```python
from build123d import *

# Parameters (mm, degrees)
F0_R     = 5
F0_R_2   = 3.15
F0_R_3   = 2.55
F1_DEPTH = 3.25
F2_R     = 2.55
F3_DEPTH = 14


# Not quite as in the source:
# - a feature names something its author has since deleted; it is built from what else it names


with BuildPart() as f1:
    # F0 (on Top) → F1 (new body)
    with BuildSketch(Plane.XY):
        with BuildLine():
            Line((-5.95, -4.4), (-4.4034787385, -4.4))
            ThreePointArc((-4.4034787385, -4.4), (0, -6.225), (4.4034787385, -4.4))
            Line((4.4034787385, -4.4), (5.95, -4.4))
            Line((5.95, -4.4), (5.95, 4.4))
            Line((5.95, 4.4), (4.4034787385, 4.4))
            ThreePointArc((4.4034787385, 4.4), (0, 6.225), (-4.4034787385, 4.4))
            Line((-4.4034787385, 4.4), (-5.95, 4.4))
            Line((-5.95, 4.4), (-5.95, -4.4))
        make_face()
        Circle(F0_R, mode=Mode.SUBTRACT)
        Circle(F0_R)
        Circle(F0_R_2, mode=Mode.SUBTRACT)
        Circle(F0_R_2)
        Circle(F0_R_3, mode=Mode.SUBTRACT)
        Circle(F0_R_3)
        with BuildLine():
            ThreePointArc((-1.275, -1.1244443072), (-0.601040764, 1.5902043894), (1.7, 0))
            ThreePointArc((1.7, 0), (1.5902043894, -0.601040764), (1.275, -1.1244443072))
            ThreePointArc((1.275, -1.1244443072), (0, -1.7), (-1.275, -1.1244443072))
        make_face(mode=Mode.SUBTRACT)
        with BuildLine():
            Line((1.275, -1.1244443072), (-1.275, -1.1244443072))
            ThreePointArc((-1.275, -1.1244443072), (0, -1.7), (1.275, -1.1244443072))
        make_face()
    extrude(amount=F1_DEPTH)

    # F2 (on face) → F3 (join)
    with BuildSketch(Plane.XY.offset(3.25)):
        with BuildLine():
            ThreePointArc((-4.8302633262, 0.3000085552), (-4.9546244936, 0.172348246), (-5, 0))
            ThreePointArc((-5, 0), (-4.9546244936, -0.172348246), (-4.8302633262, -0.3000085552))
            Line((-4.8302633262, -0.3000085552), (-4.2601369618, -0.6425750355))
            ThreePointArc((-4.2601369618, -0.6425750355), (-4.0929165173, -0.7205512094), (-3.9131380826, -0.7620563314))
            Line((-3.9131380826, -0.7620563314), (-3.3117988826, -0.835891501))
            ThreePointArc((-3.3117988826, -0.835891501), (-3.0868883315, -0.9291389359), (-2.9422567869, -1.125))
            ThreePointArc((-2.9422567869, -1.125), (-3.15, 0), (-2.9422567869, 1.125))
            ThreePointArc((-2.9422567869, 1.125), (-3.0868883315, 0.9291389359), (-3.3117988826, 0.835891501))
            Line((-3.3117988826, 0.835891501), (-3.9131380826, 0.7620563314))
            ThreePointArc((-3.9131380826, 0.7620563314), (-4.0929165173, 0.7205512094), (-4.2601369618, 0.6425750355))
            Line((-4.2601369618, 0.6425750355), (-4.8302633262, 0.3000085552))
        make_face()
        with BuildLine():
            ThreePointArc((-3.2033738691, 3.6276500367), (-3.3815799641, 3.6253171911), (-3.5355339059, 3.5355339059))
            ThreePointArc((-3.5355339059, 3.5355339059), (-3.6253171911, 3.3815799641), (-3.6276500367, 3.2033738691))
            Line((-3.6276500367, 3.2033738691), (-3.4667408995, 2.5580025694))
            ThreePointArc((-3.4667408995, 2.5580025694), (-3.4036356706, 2.3846223779), (-3.3058616735, 2.2281512744))
            Line((-3.3058616735, 2.2281512744), (-2.9328599965, 1.7507308991))
            ThreePointArc((-2.9328599965, 1.7507308991), (-2.8397601142, 1.5257592297), (-2.8759848548, 1.2849945972))
            ThreePointArc((-2.8759848548, 1.2849945972), (-2.2273863607, 2.2273863607), (-1.2849945972, 2.8759848548))
            ThreePointArc((-1.2849945972, 2.8759848548), (-1.5257592297, 2.8397601142), (-1.7507308991, 2.9328599965))
            Line((-1.7507308991, 2.9328599965), (-2.2281512744, 3.3058616735))
            ThreePointArc((-2.2281512744, 3.3058616735), (-2.3846223779, 3.4036356706), (-2.5580025694, 3.4667408995))
            Line((-2.5580025694, 3.4667408995), (-3.2033738691, 3.6276500367))
        make_face()
        with BuildLine():
            ThreePointArc((0.3000085552, 4.8302633262), (0.172348246, 4.9546244936), (0, 5))
            ThreePointArc((0, 5), (-0.172348246, 4.9546244936), (-0.3000085552, 4.8302633262))
            Line((-0.3000085552, 4.8302633262), (-0.6425750355, 4.2601369618))
            ThreePointArc((-0.6425750355, 4.2601369618), (-0.7205512094, 4.0929165173), (-0.7620563314, 3.9131380826))
            Line((-0.7620563314, 3.9131380826), (-0.835891501, 3.3117988826))
            ThreePointArc((-0.835891501, 3.3117988826), (-0.9291389359, 3.0868883315), (-1.125, 2.9422567869))
            ThreePointArc((-1.125, 2.9422567869), (0, 3.15), (1.125, 2.9422567869))
            ThreePointArc((1.125, 2.9422567869), (0.9291389359, 3.0868883315), (0.835891501, 3.3117988826))
            Line((0.835891501, 3.3117988826), (0.7620563314, 3.9131380826))
            ThreePointArc((0.7620563314, 3.9131380826), (0.7205512094, 4.0929165173), (0.6425750355, 4.2601369618))
            Line((0.6425750355, 4.2601369618), (0.3000085552, 4.8302633262))
        make_face()
        with BuildLine():
            ThreePointArc((3.2033738691, -3.6276500367), (3.3815799667, -3.6253171904), (3.5355339096, -3.5355339023))
            ThreePointArc((3.5355339096, -3.5355339023), (3.6253171918, -3.3815799616), (3.6276500367, -3.2033738691))
            Line((3.6276500367, -3.2033738691), (3.4667408995, -2.5580025694))
            ThreePointArc((3.4667408995, -2.5580025694), (3.4036356706, -2.3846223779), (3.3058616735, -2.2281512744))
            Line((3.3058616735, -2.2281512744), (2.9328599965, -1.7507308991))
            ThreePointArc((2.9328599965, -1.7507308991), (2.8397601142, -1.5257592297), (2.8759848548, -1.2849945972))
            ThreePointArc((2.8759848548, -1.2849945972), (2.2273863607, -2.2273863607), (1.2849945972, -2.8759848548))
            ThreePointArc((1.2849945972, -2.8759848548), (1.5257592297, -2.8397601142), (1.7507308991, -2.9328599965))
            Line((1.7507308991, -2.9328599965), (2.2281512744, -3.3058616735))
            ThreePointArc((2.2281512744, -3.3058616735), (2.3846223779, -3.4036356706), (2.5580025694, -3.4667408995))
            Line((2.5580025694, -3.4667408995), (3.2033738691, -3.6276500367))
        make_face()
        with BuildLine():
            ThreePointArc((-0.3000085552, -4.8302633262), (-0.172348246, -4.9546244936), (0, -5))
            ThreePointArc((0, -5), (0.172348246, -4.9546244936), (0.3000085552, -4.8302633262))
            Line((0.3000085552, -4.8302633262), (0.6425750355, -4.2601369618))
            ThreePointArc((0.6425750355, -4.2601369618), (0.7205512094, -4.0929165173), (0.7620563314, -3.9131380826))
            Line((0.7620563314, -3.9131380826), (0.835891501, -3.3117988826))
            ThreePointArc((0.835891501, -3.3117988826), (0.9291389359, -3.0868883315), (1.125, -2.9422567869))
            ThreePointArc((1.125, -2.9422567869), (0, -3.15), (-1.125, -2.9422567869))
            ThreePointArc((-1.125, -2.9422567869), (-0.9291389359, -3.0868883315), (-0.835891501, -3.3117988826))
            Line((-0.835891501, -3.3117988826), (-0.7620563314, -3.9131380826))
            ThreePointArc((-0.7620563314, -3.9131380826), (-0.7205512094, -4.0929165173), (-0.6425750355, -4.2601369618))
            Line((-0.6425750355, -4.2601369618), (-0.3000085552, -4.8302633262))
        make_face()
        with BuildLine():
            ThreePointArc((-3.6276500367, -3.2033738691), (-3.6253171911, -3.3815799641), (-3.5355339059, -3.5355339059))
            ThreePointArc((-3.5355339059, -3.5355339059), (-3.3815799641, -3.6253171911), (-3.2033738691, -3.6276500367))
            Line((-3.2033738691, -3.6276500367), (-2.5580025694, -3.4667408995))
            ThreePointArc((-2.5580025694, -3.4667408995), (-2.3846223779, -3.4036356706), (-2.2281512744, -3.3058616735))
            Line((-2.2281512744, -3.3058616735), (-1.7507308991, -2.9328599965))
            ThreePointArc((-1.7507308991, -2.9328599965), (-1.5257592297, -2.8397601142), (-1.2849945972, -2.8759848548))
            ThreePointArc((-1.2849945972, -2.8759848548), (-2.2273863607, -2.2273863607), (-2.8759848548, -1.2849945972))
            ThreePointArc((-2.8759848548, -1.2849945972), (-2.8397601142, -1.5257592297), (-2.9328599965, -1.7507308991))
            Line((-2.9328599965, -1.7507308991), (-3.3058616735, -2.2281512744))
            ThreePointArc((-3.3058616735, -2.2281512744), (-3.4036356706, -2.3846223779), (-3.4667408995, -2.5580025694))
            Line((-3.4667408995, -2.5580025694), (-3.6276500367, -3.2033738691))
        make_face()
        with BuildLine():
            ThreePointArc((2.8759848548, -1.2849945972), (2.9102205274, -1.205452812), (2.9422567869, -1.125))
            ThreePointArc((2.9422567869, -1.125), (3.0976288414, -0.5720101054), (3.15, 0))
            ThreePointArc((3.15, 0), (3.0976288414, 0.5720101054), (2.9422567869, 1.125))
            ThreePointArc((2.9422567869, 1.125), (2.9102205274, 1.205452812), (2.8759848548, 1.2849945972))
            ThreePointArc((2.8759848548, 1.2849945972), (2.2273863607, 2.2273863607), (1.2849945972, 2.8759848548))
            ThreePointArc((1.2849945972, 2.8759848548), (1.205452812, 2.9102205274), (1.125, 2.9422567869))
            ThreePointArc((1.125, 2.9422567869), (0, 3.15), (-1.125, 2.9422567869))
            ThreePointArc((-1.125, 2.9422567869), (-1.205452812, 2.9102205274), (-1.2849945972, 2.8759848548))
            ThreePointArc((-1.2849945972, 2.8759848548), (-2.2273863607, 2.2273863607), (-2.8759848548, 1.2849945972))
            ThreePointArc((-2.8759848548, 1.2849945972), (-2.9102205274, 1.205452812), (-2.9422567869, 1.125))
            ThreePointArc((-2.9422567869, 1.125), (-3.15, 0), (-2.9422567869, -1.125))
            ThreePointArc((-2.9422567869, -1.125), (-2.9102205274, -1.205452812), (-2.8759848548, -1.2849945972))
            ThreePointArc((-2.8759848548, -1.2849945972), (-2.2273863607, -2.2273863607), (-1.2849945972, -2.8759848548))
            ThreePointArc((-1.2849945972, -2.8759848548), (-1.205452812, -2.9102205274), (-1.125, -2.9422567869))
            ThreePointArc((-1.125, -2.9422567869), (0, -3.15), (1.125, -2.9422567869))
            ThreePointArc((1.125, -2.9422567869), (1.205452812, -2.9102205274), (1.2849945972, -2.8759848548))
            ThreePointArc((1.2849945972, -2.8759848548), (2.2273863607, -2.2273863607), (2.8759848548, -1.2849945972))
        make_face()
        Circle(F2_R, mode=Mode.SUBTRACT)
        Circle(F2_R)
        with BuildLine():
            Line((1.275, -1.1244443072), (-1.275, -1.1244443072))
            ThreePointArc((-1.275, -1.1244443072), (0, 1.7), (1.275, -1.1244443072))
        make_face(mode=Mode.SUBTRACT)
        with BuildLine():
            ThreePointArc((3.6276500367, 3.2033738691), (3.6253171915, 3.3815799629), (3.5355339078, 3.5355339041))
            ThreePointArc((3.5355339078, 3.5355339041), (3.3815799654, 3.6253171908), (3.2033738691, 3.6276500367))
            Line((3.2033738691, 3.6276500367), (2.5580025694, 3.4667408995))
            ThreePointArc((2.5580025694, 3.4667408995), (2.3846223779, 3.4036356706), (2.2281512744, 3.3058616735))
            Line((2.2281512744, 3.3058616735), (1.7507308991, 2.9328599965))
            ThreePointArc((1.7507308991, 2.9328599965), (1.5257592297, 2.8397601142), (1.2849945972, 2.8759848548))
            ThreePointArc((1.2849945972, 2.8759848548), (2.2273863607, 2.2273863607), (2.8759848548, 1.2849945972))
            ThreePointArc((2.8759848548, 1.2849945972), (2.8397601142, 1.5257592297), (2.9328599965, 1.7507308991))
            Line((2.9328599965, 1.7507308991), (3.3058616735, 2.2281512744))
            ThreePointArc((3.3058616735, 2.2281512744), (3.4036356706, 2.3846223779), (3.4667408995, 2.5580025694))
            Line((3.4667408995, 2.5580025694), (3.6276500367, 3.2033738691))
        make_face()
        with BuildLine():
            ThreePointArc((4.8302633262, -0.3000085552), (4.9546244936, -0.172348246), (5, 0))
            ThreePointArc((5, 0), (4.9546244936, 0.172348246), (4.8302633262, 0.3000085552))
            Line((4.8302633262, 0.3000085552), (4.2601369618, 0.6425750355))
            ThreePointArc((4.2601369618, 0.6425750355), (4.0929165173, 0.7205512094), (3.9131380826, 0.7620563314))
            Line((3.9131380826, 0.7620563314), (3.3117988826, 0.835891501))
            ThreePointArc((3.3117988826, 0.835891501), (3.0868883315, 0.9291389359), (2.9422567869, 1.125))
            ThreePointArc((2.9422567869, 1.125), (3.0976288414, 0.5720101054), (3.15, 0))
            ThreePointArc((3.15, 0), (3.0976288414, -0.5720101054), (2.9422567869, -1.125))
            ThreePointArc((2.9422567869, -1.125), (3.0868883315, -0.9291389359), (3.3117988826, -0.835891501))
            Line((3.3117988826, -0.835891501), (3.9131380826, -0.7620563314))
            ThreePointArc((3.9131380826, -0.7620563314), (4.0929165173, -0.7205512094), (4.2601369618, -0.6425750355))
            Line((4.2601369618, -0.6425750355), (4.8302633262, -0.3000085552))
        make_face()
    extrude(amount=F3_DEPTH)


solid = f1.part
```
Geometry check sheet. Reference: the model listing, model coordinates, mm. A direction names the side the tool comes from. Round coordinates to 2 decimals unless told otherwise and drop trailing zeros. Order: outer loops, then holes, each group sorted by start corner. A loop starts at its lowest first (then second) coordinate and runs counter-clockwise, first axis right, second up. Notation, with made-up numbers: M 19,76 L 25,76 A19 ccw 25,102 Z; hole C 1,-34 d2. An arc over 180 degrees is marked long. Answer as CSV lines item,"result".
1) Sectioned sample at A-A on y = -1.5. Record the cut outline in (x, z), and give its area (3 significant figures).
Entries:
outline,"M -5.95,0 L 5.95,0 L 5.95,3.25 L 2.84,3.25 L 2.84,17.25 L -2.84,17.25 L -2.84,3.25 L -5.95,3.25 Z"
area,"118 mm2"
2) Mould release check, pull along X, two halves, no side actions. Record for faces 5 (the face through (5, -4.4, 2)), 6 (the face through (-5.95, 0, 2)), 7 (the face through (0, -1.124, 9)): +X half, -X half, draft (parallel to the pull), parting line (faces both ways), or undercut.
Entries:
face 5,"draft"
face 6,"-X half"
face 7,"undercut"
3) Sectioned sample at B-B on x = 1.5. Record the cut outline in (y, z), and give its area (3 significant figures).
Entries:
outline,"M -6.04,0 L -0.8,0 L -0.8,17.25 L -2.84,17.25 L -2.84,3.25 L -6.04,3.25 Z; M 0.8,0 L 6.04,0 L 6.04,3.25 L 2.84,3.25 L 2.84,17.25 L 0.8,17.25 Z"
area,"91.1 mm2"
4) Gauge pin test, flat ends, axial feed: pin 1 Ø1.2 at (x, z) = (-5.5, 1) entering from -Y; pin 2 Ø4 at (y, z) = (-2, 11.5) entering from -X; pin 3 Ø6 at (y, z) = (-4.5, 11) entering from -X. Record the tip position at first contact, or that the pin passes through.
Entries:
pin 1,"y = -4.4"
pin 2,"x = -5"
pin 3,"x = -3.64"
5) Tool access check on faces 1 (the face through (5, 4.4, 2)), 2 (the face through (4, -1, 3.25)), 3 (the face through (-5, 4.4, 2)), 4 (the face through (-5, -4.4, 2)). Record the directions out of +Z, -Z, +X, -X, +Y, -Y that give a thin tool (end or side, any length) a straight path to the whole face; none if there is none.
Entries:
face 1,"+Z, -Z, +X, +Y"
face 2,"+Z"
face 3,"+Z, -Z, -X, +Y"
face 4,"+Z, -Z, -X, -Y"
6) Thickness scan on probe 1 along Y at (x, z) = (0, 2.35) (3 decimals); probe 2 along Y at (x, z) = (-3.25, 9); probe 3 along Z at (x, y) = (5.25, 0.25). Record the ranges inside material, lowest first. Write a range as [from, to].
Entries:
probe 1,"[-6.225, -1.124], [1.7, 6.225]"
probe 2,"[-3.64, -2.16], [-0.85, 0.85], [2.16, 3.64]"
probe 3,"[0, 3.25]"
